Autodesk Inventor part; units mm, degrees
ref_plane "YZ Plane" through (0, 0, 0) normal (1, 0, 0) x (0, 1, 0)
ref_plane "XZ Plane" through (0, 0, 0) normal (0, 1, 0) x (-1, 0, 0)
ref_plane "XY Plane" through (0, 0, 0) normal (0, 0, 1) x (1, 0, 0)
sketch "Sketch1" plane through (0, 0, 0) normal (0, 1, 0) x (-1, 0, 0)
  line L0 (0, 0) -> (-20, 0)
  line L1 (-20, 0) -> (-20, -20)
  line L2 (-20, -20) -> (0, -20)
  line L3 (0, -20) -> (0, 0)
  dimension "d0" = 20
  dimension "d1" = 20
extrude "Extrusion1" add sketch "Sketch1" along normal blind 500
sketch "Sketch2" plane through (0, 0, 0) normal (0, -1, 0) x (1, 0, 0)
  line L0 (0, 0) -> (20, 0)
  line L1 (20, 0) -> (20, -20)
  point P0 (10, -10)
  point P1 (10, 0)
  point P2 (20, -10)
hole "Hole1" at (10, 0, -10) direction (0, 1, 0) diameter 3.4 end through all
equation "\"d0\" = extrusion_dim"
equation "\"d1\" = extrusion_dim"
equation "\"d2\" = tower_height"
equation "\"base_thickness\" = 12.7"
equation "\"tower_height\" = 500"
equation "\"extrusion_dim\" = 20"
equation "\"top_sheet_thickness\" = 6.35"
properties part number "Tower" material "Aluminum 6061"
The listing builds one solid part. Answer for the finished solid, in the listing's coordinates (mm). Coordinates: 2 decimals unless noted, no trailing zeros. Loops run counter-clockwise (first coordinate to the right, second up) from the corner with the lowest first, then second, coordinate; pieces in that order, holes last. Notation, with made-up numbers: (59.25, 38) - (89.25, 38) arc R15 cw to (89.25, 43) - close; hole circle Ø11 at (38, 25). An arc over 180 degrees is marked (long way). Use a Markdown table: item, result. Add a question column.
1) The mould has two halves that part along Z. Classify faces 1 (the flat face through (20, 246, -10)), 2 (the flat face through (10, 246, -20)), 3 (the flat face through (10, 246, 0)): released by +Z, released by -Z, zero draft, split by the parting line, or undercut.
2) Given pin 1 (10 mm diameter, centred on x = 12, z = -10.5, fed in from -Y); pin 2 (2 mm diameter, centred on x = 10, z = -10, fed in from -Y), each flat-ended and moving along its own axis, determine where each tip first touches the part or whether it passes through.
3) The part is cut by section A-A, the plane y = 108. Give the vertices of the cut face in (x, z), and give its area (3 significant figures).
4) Find the intervals of material crossed by line 1 (Z direction, x = 10, y = 195); line 2 (X direction, y = 323.5, z = -10); line 3 (X direction, y = 83, z = -9.5), in increasing order.
Here are the results:
| question | item | result |
|---|---|---|
| 1 | face 1 | zero draft |
| 1 | face 2 | released by -Z |
| 1 | face 3 | released by +Z |
| 2 | pin 1 | stops at y = 0 |
| 2 | pin 2 | passes through |
| 3 | outline | (0, -20) - (20, -20) - (20, 0) - (0, 0) - close; hole circle Ø3.4 at (10, -10) |
| 3 | area | 391 mm^2 |
| 4 | line 1 | z = -20 to -11.7, -8.3 to 0 |
| 4 | line 2 | x = 0 to 8.3, 11.7 to 20 |
| 4 | line 3 | x = 0 to 8.38, 11.62 to 20 |
